Can you work these out from the drawing? Everything is in mm from the part's minimum corner. A direction names the side the tool comes from. Give positions to 0.01 mm unless a question says otherwise; leave off trailing zeros. Order: outer loops, then holes, each group sorted by start corner. A loop starts at its lowest first (then second) coordinate and runs counter-clockwise, first axis right, second up. Notation, with made-up numbers: (-30.5, 65) -> (26.5, 65) arc R23 ccw to (26.5, 89) -> close; hole circle Ø11 at (-16.5, 87). An arc over 180 degrees is marked (long way). One line per item, written item: value.
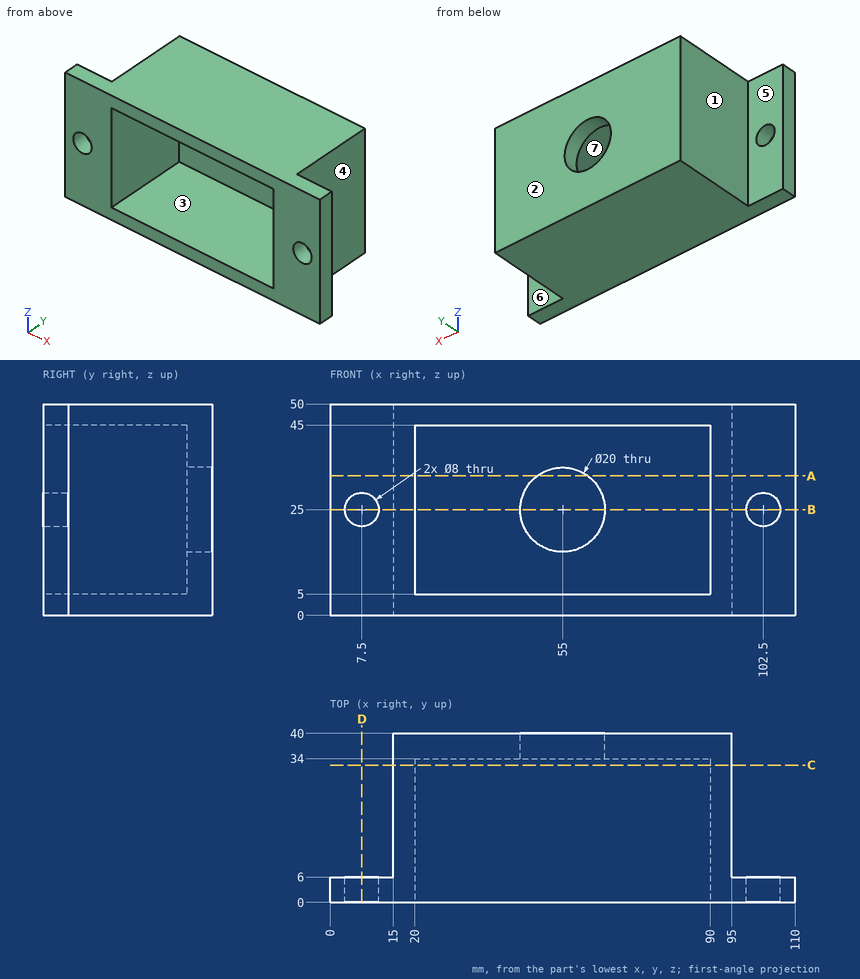
1) Suppose I cut it at A-A, the plane z = 33. Write out the boundary of the cut face in (x, y).
Answer below:
outline: (0, 0) -> (20, 0) -> (20, 34) -> (49, 34) -> (49, 40) -> (15, 40) -> (15, 6) -> (0, 6) -> close; (61, 34) -> (90, 34) -> (90, 0) -> (110, 0) -> (110, 6) -> (95, 6) -> (95, 40) -> (61, 40) -> close
2) If I drill on line 1 along X through (y, z) = (4, 25); line 2 along Z through (x, y) = (61, 7.5); line 3 along X through (y, z) = (17.5, 18), over which ranges is the centre line in solid material (lowest first)?
Answer below:
line 1: x = 0 to 3.5, 11.5 to 20, 90 to 98.5, 106.5 to 110
line 2: z = 0 to 5, 45 to 50
line 3: x = 15 to 20, 90 to 95
3) Suppose I cut it at B-B, the plane z = 25. Write out the boundary of the cut face in (x, y), then the cut area to 3 significant figures.
Answer below:
outline: (0, 0) -> (3.5, 0) -> (3.5, 6) -> (0, 6) -> close; (11.5, 0) -> (20, 0) -> (20, 34) -> (45, 34) -> (45, 40) -> (15, 40) -> (15, 6) -> (11.5, 6) -> close; (65, 34) -> (90, 34) -> (90, 0) -> (98.5, 0) -> (98.5, 6) -> (95, 6) -> (95, 40) -> (65, 40) -> close; (106.5, 0) -> (110, 0) -> (110, 6) -> (106.5, 6) -> close
area: 784 mm2
4) For the marked faces 5, 6 and 7, which set-ups out of +Z, -Z, +X, -X, +Y, -Y let a thin tool reach every point of the face, with its end or its side?
Answer below:
face 5: +Z, -Z, -X, +Y
face 6: +Z, -Z, +X, +Y
face 7: -Y
5) We'd pull the mould along X, two halves only. Please class the marked faces 1, 2, 3 and 4: +X half, -X half, draft (parallel to the pull), parting line (faces both ways), or undercut.
Answer below:
face 1: -X half
face 2: draft
face 3: undercut
face 4: +X half
6) Suppose I cut it at D-D, the plane x = 7.5. Write out the boundary of the cut face in (y, z), then the cut area to 3 significant figures.
Answer below:
outline: (0, 0) -> (6, 0) -> (6, 21) -> (0, 21) -> close; (0, 29) -> (6, 29) -> (6, 50) -> (0, 50) -> close
area: 252 mm2
7) Suppose I cut it at C-C, the plane y = 32.5. Write out the boundary of the cut face in (x, z).
Answer below:
outline: (15, 0) -> (95, 0) -> (95, 50) -> (15, 50) -> close; hole (20, 5) -> (90, 5) -> (90, 45) -> (20, 45) -> close
8) For P1, Ø3, axis at x = 80, z = 12, coming from the -Y side; P2, Ø17, axis at y = 15, z = 19, coming from the +X side; P3, Ø7.5, axis at x = 10, z = 14.5, coming from the +Y side, each with a flat end and sliding along its axis, tell me the tip position at first contact or that it passes through.
Answer below:
P1: stops at y = 34
P2: stops at x = 95
P3: stops at y = 6
